Check sheet for the modelled part. Datum: model origin and axes. Units: mm. Round coordinates to 2 decimals unless told otherwise and drop trailing zeros. Write each loop counter-clockwise with the first axis right and the second up, starting at its lowest first coordinate (ties: lowest second). Pieces come first, ordered by that corner, then holes. Notation, with made-up numbers: (-12.75, 65) - (26.25, 65) arc R17 ccw to (26.25, 93) - close; hole circle Ø5 at (55.5, 76.25). An arc over 180 degrees is marked (long way). Answer as a JSON object with one key per item and string values. Group by question number.
Item 1: Sectioned sample at C-C on z = 2.1. Record the boundary of the cut face in (x, y).
Item 2: Sectioned sample at D-D on y = -11.3. Count the separate pieces of the cut face and the enclosed holes in it, plus the area to 3 significant figures.
Item 3: Gauge pin test, flat ends, axial feed: P1, Ø6, axis at x = 3.5, y = 6.5, coming from the -Z side; P2, Ø3, axis at x = 0, y = 22.6, coming from the -Z side; P3, Ø1.8, axis at x = -19.57, y = -11.3, coming from the +Z side; P4, Ø1, axis at x = 2, z = 2, coming from the +Y side. Record the tip position at first contact, or that the pin passes through.
Item 4: Thickness scan on line 1 (X direction, y = 10, z = 0.55); line 2 (Y direction, x = 0, z = 1.9); line 3 (Y direction, x = -0.5, z = 1.85). Record the ranges inside material, lowest first.
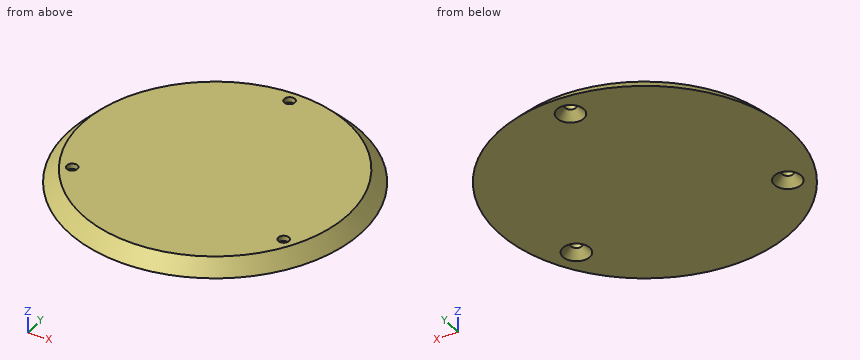
Autodesk Inventor part; units mm, degrees
ref_plane "YZ Plane" through (0, 0, 0) normal (1, 0, 0) x (0, 1, 0)
ref_plane "XZ Plane" through (0, 0, 0) normal (0, 1, 0) x (-1, 0, 0)
ref_plane "XY Plane" through (0, 0, 0) normal (0, 0, 1) x (1, 0, 0)
sketch "Esboço1" plane through (0, 0, 0) normal (0, 0, 1) x (1, 0, 0)
  circle A0 centre (0, 0) radius 27.2
  circle A1 centre (0, 22.6) radius 1
  circle A2 centre (-19.5722, -11.3) radius 1
  circle A3 centre (0, 0) radius 27.2
  circle A4 centre (19.5722, -11.3) radius 1
  circle A5 centre (0, 0) radius 27.2
  dimension "d8" = 360
  dimension "d18" = 22.6
  dimension "d19" = 54.4
extrude "Extrusão1" add sketch "Esboço1" along normal blind 2.5
chamfer "Chanfro1" distance 2.5 angle 45 1 edges at (-27.2, 0, 2.5)
chamfer "Chanfro2" distance 1.5 angle 45 3 edges at (18.5722, -11.3, 0) (-20.5722, -11.3, 0) (-1, 22.6, 0)
properties part number "Tampa inferior"
Completed:
{
 "1": {"outline": "circle Ø50.2 at (0, 0); hole circle Ø2 at (-19.57, -11.3); hole circle Ø2 at (0, 22.6); hole circle Ø2 at (19.57, -11.3)"},
 "2": {"separate pieces": "3", "enclosed holes": "0", "area": "102 mm²"},
 "3": {"P1": "z = 0", "P2": "z = 1", "P3": "through", "P4": "y = 25.62"},
 "4": {"line 1": "-24.7 to 24.7", "line 2": "-25.3 to 21.6, 23.6 to 25.3", "line 3": "-25.35 to 21.73, 23.47 to 25.35"}
}
